Can you work these out from the model? Positions are in its coordinate system, mm. A direction names the side the tool comes from. Coordinates: 2 decimals unless noted, no trailing zeros. Write item = value, one per line. Start each with the question number.
from build123d import *

# Parameters (mm, degrees)
F1_DEPTH = 25
F1_TAPER = -10
F2_T     = -2
F3_R     = 1.5
F4_DEPTH = 25


with BuildPart() as f1:
    # F0 (on Top) → F1 (new body)
    with BuildSketch(Plane.XY):
        Polygon((0, 13), (0, 0), (8, 0), (13, 0), (27, 0), (32, 0), (40, 0), (40, 13), (40, 21), (40, 34), (32, 34), (27, 34), (13, 34), (8, 34), (0, 34), (0, 21), align=None)
    extrude(amount=F1_DEPTH, taper=F1_TAPER)

    # F2
    f2_openings = [f1.faces().sort_by_distance(p)[0] for p in [
        (20, 17, 25),
    ]]
    offset(amount=F2_T, openings=f2_openings)

    # F3 (on face) → F4 (cut)
    with BuildSketch(Plane.XY.offset(2)):
        with Locations((20, 17)):
            Circle(F3_R)
    extrude(amount=-F4_DEPTH, mode=Mode.SUBTRACT)


solid = f1.part
(1) If I drill on L1, parallel to Z at x = 18, y = 2; L2, parallel to Y at x = 3, z = 13.5; L3, parallel to Y at x = 3.5, z = 23, over which ranges is the centre line in solid material (lowest first)? Write a range as from..to.
(2) For P1, Ø15.5, axis at x = 20, y = 14.5, coming from the +Z side; P2, Ø6, axis at x = 28.5, z = 21, coming from the +Y side; P3, Ø2, axis at y = 10, z = 6.5, coming from the +X side; P4, Ø2.5, axis at x = 20, y = 17, coming from the +Z side, each with a flat end and sliding along its axis, tell me the tip position at first contact or that it passes through.
(3) For faces 1 (the face through (21, 37, 25)), 2 (the face through (-0.378, 17.271, 13.661)), which set-ups out of +Z, -Z, +X, -X, +Y, -Y let a thin tool reach every point of the face, with its end or its side?
(4) Thinking about a two-plate mould opening in X: for faces 3 (the face through (16, 21, 0)), 4 (the face through (40.378, 16.729, 13.661)), which applies, +X half, -X half, draft (parallel to the pull), parting line (faces both ways), or undercut?
Result set:
q1.L1 = 0..2
q1.L2 = -2.38..-0.35, 34.35..36.38
q1.L3 = -4.06..-2.02, 36.02..38.06
q2.P1 = 2
q2.P2 = 38.23
q2.P3 = 41.32
q2.P4 = through
q3.face_1 = +Z, +X, -X, +Y, -Y
q3.face_2 = +Z
q4.face_3 = draft
q4.face_4 = undercut
